Source: three-view drawing plus pictorial views. Frame: mm from the lowest corner of the part. A direction names the side the tool comes from. Round coordinates to 2 decimals unless told otherwise and drop trailing zeros. Write each loop counter-clockwise with the first axis right and the second up, starting at its lowest first coordinate (ties: lowest second). Pieces come first, ordered by that corner, then holes. Notation, with made-up numbers: (-28.5, 86.5) -> (16.5, 86.5) arc R20 ccw to (16.5, 98.5) -> close; hole circle Ø9 at (-33.5, -34). An arc over 180 degrees is marked (long way). Put each result on its own line as item: value.
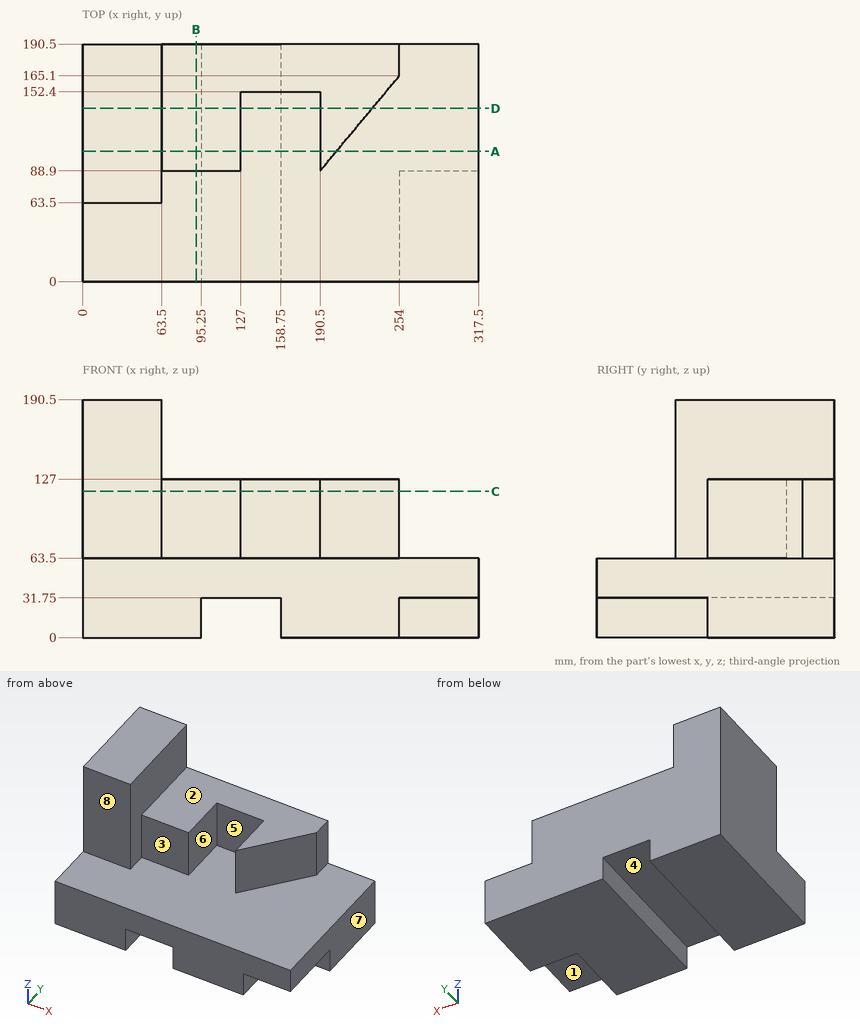
Q1. Cut plane D-D on y = 139. Output: boundary loops of the cut face in (x, z), and give its area (3 significant figures).
Ans:
outline: (0, 0) -> (95.25, 0) -> (95.25, 31.75) -> (158.75, 31.75) -> (158.75, 0) -> (317.5, 0) -> (317.5, 63.5) -> (232.25, 63.5) -> (232.25, 127) -> (190.5, 127) -> (190.5, 63.5) -> (127, 63.5) -> (127, 127) -> (63.5, 127) -> (63.5, 190.5) -> (0, 190.5) -> close
area: 32,900 mm^2
Q2. Cut plane A-A on y = 104.5. Output: boundary loops of the cut face in (x, z), and give its area (3 significant figures).
Ans:
outline: (0, 0) -> (95.25, 0) -> (95.25, 31.75) -> (158.75, 31.75) -> (158.75, 0) -> (317.5, 0) -> (317.5, 63.5) -> (203.5, 63.5) -> (203.5, 127) -> (190.5, 127) -> (190.5, 63.5) -> (127, 63.5) -> (127, 127) -> (63.5, 127) -> (63.5, 190.5) -> (0, 190.5) -> close
area: 31,100 mm^2
Q3. Reachability of the marked faces 1, 2, 3 and 4 from +Z, -Z, +X, -X, +Y, -Y: full face, straight path, thin tool, end or side. Return the list, or none.
Ans:
face 1: -Z, +X, -Y
face 2: +Z, +X, +Y, -Y
face 3: +Z, +X, -Y
face 4: -Z, +Y, -Y
Q4. Cut plane B-B on x = 91. Output: boundary loops of the cut face in (y, z).
Ans:
outline: (0, 0) -> (190.5, 0) -> (190.5, 127) -> (88.9, 127) -> (88.9, 63.5) -> (0, 63.5) -> close
Q5. Draft query along X for the marked faces 5, 6, 7 and 8. Return one class per face: +X half, -X half, draft (parallel to the pull), parting line (faces both ways), or undercut.
Ans:
face 5: undercut
face 6: undercut
face 7: +X half
face 8: draft
Q6. Material intervals for line 1 (X direction, y = 110, z = 28.5); line 2 (X direction, y = 86.5, z = 11.5); line 3 (Z direction, x = 265.5, y = 88.5), sorted ascending. Write a range as [from, to].
Ans:
line 1: x = [0, 95.25], [158.75, 317.5]
line 2: x = [0, 95.25], [158.75, 254]
line 3: z = [31.75, 63.5]
Q7. Cut plane C-C on z = 117. Output: boundary loops of the cut face in (x, y), and give its area (3 significant figures).
Ans:
outline: (0, 63.5) -> (63.5, 63.5) -> (63.5, 88.9) -> (127, 88.9) -> (127, 152.4) -> (190.5, 152.4) -> (190.5, 88.9) -> (254, 165.1) -> (254, 190.5) -> (0, 190.5) -> close
area: 21,000 mm^2
Q8. Pin query (flat end, axial travel): pin 1 (12 mm diameter, centred on x = 66.5, z = 100.5, fed in from -Y); pin 2 (3 mm diameter, centred on y = 73.5, z = 153.5, fed in from +X); pin 3 (16 mm diameter, centred on y = 42.5, z = 20.5, fed in from +X). Return the tip coordinate at first contact, or that it passes through.
Ans:
pin 1: stops at y = 63.5
pin 2: stops at x = 63.5
pin 3: stops at x = 254
